from build123d import *

# Parameters (mm, degrees)
SKETCH2_R           = 1.27
SKETCH2_R_2         = 3.175
BOSS_EXTRUDE1_DEPTH = 4


with BuildPart() as part:
    # Sketch2 → Boss-Extrude1 (new body)
    with BuildSketch(Plane.XY):
        with BuildLine():
            Line((4.552043366, 53.654489758), (6.242956634, 98.745510242))
            ThreePointArc((6.242956634, 98.745510242), (6.323236809, 101.600501634), (6.35, 104.456496116))
            Line((6.35, 104.456496116), (6.35, 149.86))
            ThreePointArc((6.35, 149.86), (5.606051224, 151.656051224), (3.81, 152.4))
            Line((3.81, 152.4), (-3.81, 152.4))
            ThreePointArc((-3.81, 152.4), (-5.606051224, 151.656051224), (-6.35, 149.86))
            Line((-6.35, 149.86), (-6.35, 104.456496116))
            ThreePointArc((-6.35, 104.456496116), (-6.323236809, 101.600501634), (-6.242956634, 98.745510242))
            Line((-6.242956634, 98.745510242), (-4.552043366, 53.654489758))
            ThreePointArc((-4.552043366, 53.654489758), (-4.471763191, 50.799498366), (-4.445, 47.943503884))
            Line((-4.445, 47.943503884), (-4.445, -36.540821929))
            ThreePointArc((-4.445, -36.540821929), (-5.702774085, -46.249600926), (-9.393051948, -55.317358893))
            ThreePointArc((-9.393051948, -55.317358893), (0, -71.432377699), (9.393051948, -55.317358893))
            ThreePointArc((9.393051948, -55.317358893), (5.702774085, -46.249600926), (4.445, -36.540821929))
            Line((4.445, -36.540821929), (4.445, 47.943503884))
            ThreePointArc((4.445, 47.943503884), (4.471763191, 50.799498366), (4.552043366, 53.654489758))
        make_face()
        with Locations((0, 143.51)):
            Circle(SKETCH2_R, mode=Mode.SUBTRACT)
        with Locations((0, -60.637377699)):
            Circle(SKETCH2_R_2, mode=Mode.SUBTRACT)
    extrude(amount=BOSS_EXTRUDE1_DEPTH)


solid = part.part
Geometry check sheet. Reference: the model listing, model coordinates, mm. A direction names the side the tool comes from. Coordinates: 2 decimals unless noted, no trailing zeros. Write each loop counter-clockwise with the first axis right and the second up, starting at its lowest first coordinate (ties: lowest second). Pieces come first, ordered by that corner, then holes. Notation, with made-up numbers: (-2, 23.5) -> (7, 23.5) arc R22 ccw to (7, 36.5) -> close; hole circle Ø6 at (-34, 26). An arc over 180 degrees is marked (long way). One line per question, with ' | ' between items.
1. Depth check by flat-ended pin: pin 1 Ø1.2 at (y, z) = (128, 1.5) entering from -X; pin 2 Ø4 at (x, y) = (0, -60.64) entering from +Z; pin 3 Ø1.5 at (x, y) = (5.5, 116.5) entering from -Z; pin 4 Ø2 at (y, z) = (120.5, 2.5) entering from +X. Enter the tip coordinate at first touch or a pass-through.
Answers:
pin 1: stops at x = -6.35 | pin 2: passes through | pin 3: stops at z = 0 | pin 4: stops at x = 6.35
2. Cross-section at C-C on y = 93. Record the cut outline in (x, z), and give its area (3 significant figures).
Answers:
outline: (-6.03, 0) -> (6.03, 0) -> (6.03, 4) -> (-6.03, 4) -> close | area: 48.2 mm²
3. Draft check along Y on faces 1 (the cylindrical face through (-4.473, 50.839, 1.972)), 2 (the flat face through (0, 42, 0)), 3 (the cylindrical face through (-0.315, -71.428, 1.972)). Enter one of: +Y half, -Y half, draft (parallel to the pull), parting line (faces both ways), or undercut.
Answers:
face 1: undercut | face 2: draft | face 3: parting line
4. Cross-section at B-B on y = -30.5. Record the cut outline in (x, z) (3 decimals).
Answers:
outline: (-4.445, 0) -> (4.445, 0) -> (4.445, 4) -> (-4.445, 4) -> close
5. Cross-section at A-A on z = 1.5. State how many separate pieces and enclosed holes the cut face has, and give its area (3 significant figures).
Answers:
separate pieces: 1 | enclosed holes: 2 | area: 2,450 mm²
6. Thickness scan on probe 1 along X at (y, z) = (138, 2.15); probe 2 along X at (y, z) = (11, 0.7) (3 decimals); probe 3 along Y at (x, z) = (-2.25, 3.35). Record the ranges inside material, lowest first. Write a range as from..to.
Answers:
probe 1: x = -6.35..6.35 | probe 2: x = -4.445..4.445 | probe 3: y = -71.2..-62.88, -58.4..152.4
7. Set-up check for faces 4 (the flat face through (6.35, 127, 2)), 5 (the flat face through (-5.41, 76.52, 1.97)): record each of +Z, -Z, +X, -X, +Y, -Y from which the full face is reachable in a straight line by a thin tool's end or side.
Answers:
face 4: +Z, -Z, +X, +Y | face 5: +Z, -Z, -X
